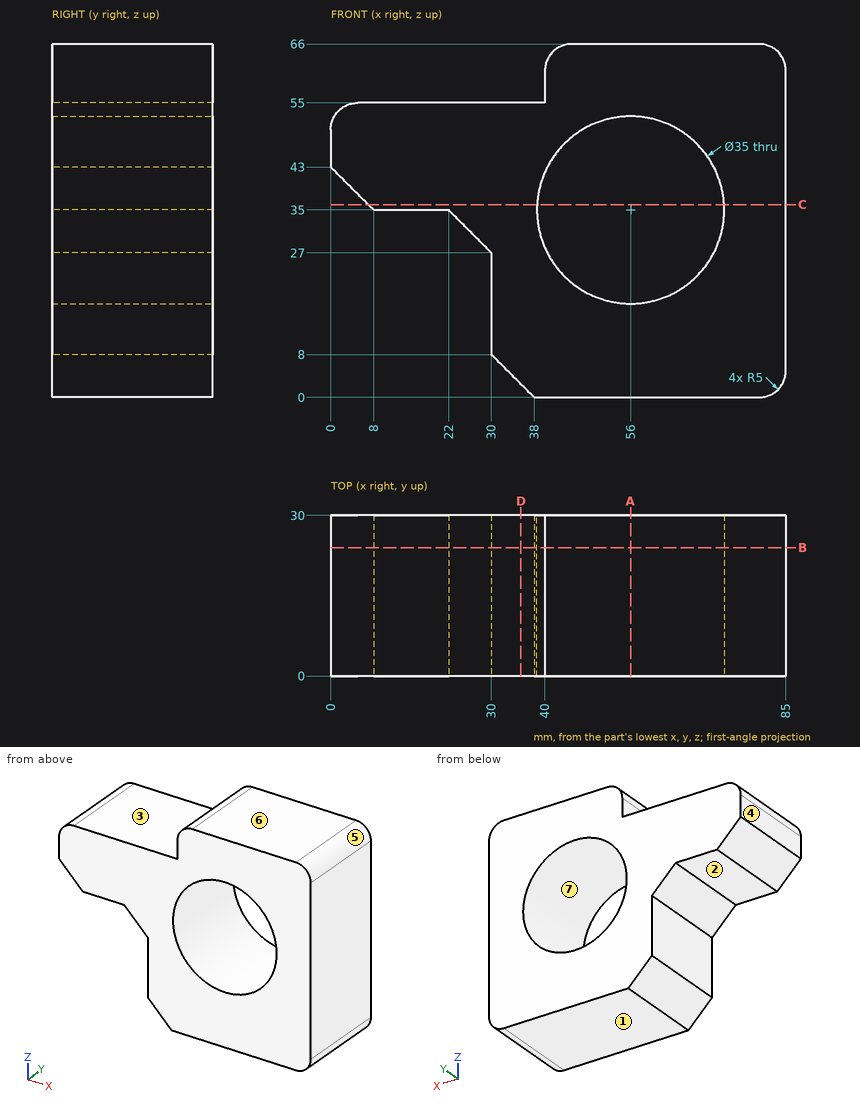
Check sheet for the drawn part. Datum: minimum x, y, z corner. Units: mm. A direction names the side the tool comes from. Coordinates: 2 decimals unless noted, no trailing zeros. Order: outer loops, then holes, each group sorted by start corner. A loop starts at its lowest first (then second) coordinate and runs counter-clockwise, first axis right, second up. Notation, with made-up numbers: M 21.25,27 L 66.25,27 A23 ccw 66.25,59 Z; hole C -25,57.25 d6. An arc over 180 degrees is marked long. One line per item, written item: value. Start each with the question number.
Item 1: Gauge pin test, flat ends, axial feed: pin 1 (3 mm diameter, centred on y = 22.5, z = 59.5, fed in from -X); pin 2 (12 mm diameter, centred on x = 35.5, y = 23.5, fed in from -Z); pin 3 (7 mm diameter, centred on x = 16.5, y = 17.5, fed in from -Z); pin 4 (15 mm diameter, centred on y = 11.5, z = 16, fed in from -X). Record the tip position at first contact, or that the pin passes through.
Item 2: Sectioned sample at A-A (x = 56). Enter the section's corners in (y, z), then the cut area to 3 significant figures.
Item 3: Sectioned sample at C-C (z = 36). Enter the section's corners in (x, y), then the cut area to 3 significant figures.
Item 4: Sectioned sample at B-B (y = 24). Enter the section's corners in (x, z).
Item 5: Mould release check, pull along X, two halves, no side actions. Record for the marked faces 4, 5, 6 and 7: released by +X, released by -X, zero draft, split by the parting line, or undercut.
Item 6: Access from +Z, -Z, +X, -X, +Y, -Y to the whole of each face (thin tool, end or side, straight path). Record for the marked faces 1, 2 and 3.
Item 7: Sectioned sample at D-D (x = 35.5). Enter the section's corners in (y, z), then the cut area to 4 significant figures.
Item 8: Scan lines: probe 1 along Z at (x, y) = (56, 22.5); probe 2 along X at (y, z) = (4.5, 43.5); probe 3 along Z at (x, y) = (65.5, 27.5). Record each from-to range of solid material in increasing order.
Conclusion:
1. pin 1: stops at x = 40
1. pin 2: stops at z = 0
1. pin 3: stops at z = 35
1. pin 4: stops at x = 30
2. outline: M 0,0 L 30,0 L 30,17.5 L 0,17.5 Z; M 0,52.5 L 30,52.5 L 30,66 L 0,66 Z
2. area: 930 mm^2
3. outline: M 7,0 L 38.53,0 L 38.53,30 L 7,30 Z; M 73.47,0 L 85,0 L 85,30 L 73.47,30 Z
3. area: 1,290 mm^2
4. outline: M 0,43 L 8,35 L 22,35 L 30,27 L 30,8 L 38,0 L 80,0 A5 ccw 85,5 L 85,61 A5 ccw 80,66 L 45,66 A5 ccw 40,61 L 40,55 L 5,55 A5 ccw 0,50 Z; hole C 56,35 d35
5. face 4: released by -X
5. face 5: released by +X
5. face 6: zero draft
5. face 7: undercut
6. face 1: -Z, +X, -X, +Y, -Y
6. face 2: -Z, -X, +Y, -Y
6. face 3: +Z, -X, +Y, -Y
7. outline: M 0,2.5 L 30,2.5 L 30,55 L 0,55 Z
7. area: 1,575 mm^2
8. probe 1: z = 0 to 17.5, 52.5 to 66
8. probe 2: x = 0 to 40.7, 71.3 to 85
8. probe 3: z = 0 to 20.3, 49.7 to 66
